Part model, mm, in its own coordinate system. A direction names the side the tool comes from. Round coordinates to 2 decimals unless told otherwise and drop trailing zeros. Write each loop counter-clockwise with the first axis right and the second up, starting at its lowest first coordinate (ties: lowest second). Pieces come first, ordered by that corner, then holes. Notation, with made-up numbers: (85.5, 12.5) -> (96.5, 12.5) arc R12 ccw to (96.5, 31.5) -> close; hole circle Ø4 at (21, 83.5). An arc over 180 degrees is marked (long way). Return JSON: item names as keys, results as strings. Group by question number.
(1) Tool access for faces 1 (the flat face through (2, 10.5, 0)), 2 (the flat face through (0, 10.5, -2)), 3 (the flat face through (0, 6, 1.5)): list every direction of +Z, -Z, +X, -X, +Y, -Y with a clear straight run to the whole face (end or side of a thin tool).
(2) Saw through at B-B (z = -1.8). List the corners of the cut face in (x, y).
(3) Saw through at D-D (z = 1.1). List the corners of the cut face in (x, y).
(4) Saw through at C-C (y = 9.25). List the corners of the cut face in (x, z), plus the area to 3 significant figures.
(5) Drill centre lines: L1, parallel to Z at x = 1.3, y = 4.75; L2, parallel to Z at x = 0, y = 10.25. Where is each one in solid material? Low to high. Write a range as from..to.
(6) Drop flat-ended pins along their axis: pin 1 Ø0.8 at (y, z) = (10.5, 0.5) entering from +X; pin 2 Ø0.9 at (x, z) = (0.5, 0.5) entering from +Y; pin 3 Ø0.5 at (y, z) = (10.5, 0) entering from -X. Give the stop position or say it passes through.
(7) Saw through at A-A (x = 0.3). List the corners of the cut face in (y, z).
(8) Mould opens along X. For faces 4 (the flat face through (0, 6, -1.5)), 5 (the flat face through (-2, 10.5, 0)), 6 (the flat face through (0, 10.5, 2)) say: +X half, -X half, draft (parallel to the pull), parting line (faces both ways), or undercut.
Autodesk Inventor part; units mm, degrees
ref_plane "YZ Plane" through (0, 0, 0) normal (1, 0, 0) x (0, 1, 0)
ref_plane "XZ Plane" through (0, 0, 0) normal (0, 1, 0) x (-1, 0, 0)
ref_plane "XY Plane" through (0, 0, 0) normal (0, 0, 1) x (1, 0, 0)
sketch "Sketch1" plane through (0, 0, 0) normal (0, 1, 0) x (-1, 0, 0)
  line L0 (-2.5, 2.5) -> (2.5, 2.5)
  line L1 (2.5, 2.5) -> (2.5, -2.5)
  line L2 (2.5, -2.5) -> (-2.5, -2.5)
  line L3 (-2.5, -2.5) -> (-2.5, 2.5)
  line L4 (-2.5, 2.5) -> (2.5, -2.5) construction
  line L5 (2.5, 2.5) -> (-2.5, -2.5) construction
  point P0 (0, 0)
  dimension "d0" = 5
  dimension "d1" = 5
extrude "Extrusion1" add sketch "Sketch1" along normal blind 10
shell "Shell1" thickness 1 removed faces 1 at (-0.8333, 10, -0.8333)
sketch "Sketch2" plane through (0, 10, 0) normal (0, 1, 0) x (1, 0, 0)
  line L0 (1.5, 1.5) -> (1.5, -1.5)
  line L1 (1.5, -1.5) -> (-1.5, -1.5)
  line L2 (-1.5, -1.5) -> (-1.5, 1.5)
  line L3 (-1.5, 1.5) -> (1.5, 1.5)
  line L4 (2.5, 2.5) -> (-2.5, 2.5)
  line L5 (-2.5, 2.5) -> (-2.5, -2.5)
  line L6 (-2.5, -2.5) -> (2.5, -2.5)
  line L7 (2.5, -2.5) -> (2.5, 2.5)
  line L8 (-2, 2) -> (-2, -2)
  line L9 (-2, -2) -> (2, -2)
  line L10 (2, -2) -> (2, 2)
  line L11 (2, 2) -> (-2, 2)
  point P0 (0, 0)
  dimension "d5" = 0.5
extrude "Extrusion2" add sketch "Sketch2" along normal blind 1 contours L11 L10 L9 L8
properties part number "snapfit_v02"
Computed values:
{
 "1": {"face 1": "+Z, -Z, +X, +Y", "face 2": "-Z, +X, -X, +Y", "face 3": "+Y"},
 "2": {"outline": "(-2.5, 0) -> (2.5, 0) -> (2.5, 10) -> (2, 10) -> (2, 11) -> (-2, 11) -> (-2, 10) -> (-2.5, 10) -> close"},
 "3": {"outline": "(-2.5, 0) -> (2.5, 0) -> (2.5, 10) -> (2, 10) -> (2, 11) -> (1.5, 11) -> (1.5, 1) -> (-1.5, 1) -> (-1.5, 11) -> (-2, 11) -> (-2, 10) -> (-2.5, 10) -> close"},
 "4": {"outline": "(-2.5, -2.5) -> (2.5, -2.5) -> (2.5, 2.5) -> (-2.5, 2.5) -> close; hole (-1.5, -1.5) -> (1.5, -1.5) -> (1.5, 1.5) -> (-1.5, 1.5) -> close", "area": "16.0 mm2"},
 "5": {"L1": "-2.5..-1.5, 1.5..2.5", "L2": "-2..-1.5, 1.5..2"},
 "6": {"pin 1": "x = 2", "pin 2": "y = 1", "pin 3": "x = -2"},
 "7": {"outline": "(0, -2.5) -> (10, -2.5) -> (10, -2) -> (11, -2) -> (11, -1.5) -> (1, -1.5) -> (1, 1.5) -> (11, 1.5) -> (11, 2) -> (10, 2) -> (10, 2.5) -> (0, 2.5) -> close"},
 "8": {"face 4": "undercut", "face 5": "-X half", "face 6": "draft"}
}
